```python
from build123d import *

# Parameters (mm, degrees)
SKETCH_1_R          = 2.1
SKETCH_1_R_2        = 4
SKETCH_1_R_3        = 11
EXTRUDE_1_DEPTH     = 3
SKETCH_3_R          = 2.1
CUT_EXTRUDE_1_DEPTH = 99.947101842
CHAMFER_2_SIZE      = 4
CHAMFER_3_SIZE      = 10
CHAMFER_3_SIZE2     = 7.354021529
SKETCH_4_W          = 7.6
SKETCH_4_H          = 9.2
CUT_EXTRUDE_2_DEPTH = 97.00692173
FILLET_1_R          = 2
SKETCH_5_R          = 2.1
CUT_EXTRUDE_3_DEPTH = 97.00692173
CHAMFER_1_SIZE      = 2
SKETCH_6_R          = 35
CUT_EXTRUDE_4_DEPTH = 97.00692173
FILLET_START        = -3
FILLET_2_DEPTH      = 6
CHAMFER_4_SIZE      = 4


with BuildPart() as part:
    # 草图1 → 凸台-拉伸1 (new, symmetric)
    with BuildSketch(Plane.XY):
        with BuildLine():
            Line((-55, 82.03370626), (-55, -2.96629374))
            Line((-55, -2.96629374), (-34.874074919, -2.96629374))
            ThreePointArc((-34.874074919, -2.96629374), (-7.334524273, -34.22286887), (30.595504664, -16.997502591))
            Line((30.595504664, -16.997502591), (52.449436567, 22.339574834))
            Line((52.449436567, 22.339574834), (-55, 82.03370626))
        make_face()
        with Locations((29, 0)):
            Circle(SKETCH_1_R, mode=Mode.SUBTRACT)
        with Locations((-14.5, -25.11473671)):
            Circle(SKETCH_1_R, mode=Mode.SUBTRACT)
        with Locations((-14.5, 25.11473671)):
            Circle(SKETCH_1_R, mode=Mode.SUBTRACT)
        with Locations((-9.625, 16.670989023)):
            Circle(SKETCH_1_R_2, mode=Mode.SUBTRACT)
        Circle(SKETCH_1_R_3, mode=Mode.SUBTRACT)
    extrude(amount=EXTRUDE_1_DEPTH, both=True)

    # 草图3 → 切除-拉伸1 (cut, through all)
    with BuildSketch(Plane.XY.offset(3)):
        with Locations((-45, 7.03370626)):
            Circle(SKETCH_3_R)
        with Locations((-45, 57.03370626)):
            Circle(SKETCH_3_R)
    extrude(amount=-CUT_EXTRUDE_1_DEPTH, mode=Mode.SUBTRACT)

    # 倒角2
    chamfer_2_edges = [part.edges().sort_by_distance(p)[0] for p in [
        (52.449436567, 22.339574834, 0),
        (-55, -2.96629374, 0),
    ]]
    chamfer(chamfer_2_edges, length=CHAMFER_2_SIZE)

    # 倒角3
    chamfer_3_edges = [part.edges().sort_by_distance(p)[0] for p in [
        (-55, 82.03370626, 0),
    ]]
    chamfer_3_side = [part.faces().sort_by_distance(p)[0] for p in [
        (-55, 41.53370626, 0),
    ]]
    chamfer(chamfer_3_edges, length=CHAMFER_3_SIZE, length2=CHAMFER_3_SIZE2, reference=chamfer_3_side[0])

    # 草图4 → 切除-拉伸2 (cut, through all)
    with BuildSketch(Plane.XY.offset(3)):
        with Locations((-18.5, 0)):
            Rectangle(SKETCH_4_W, SKETCH_4_H)
    extrude(amount=-CUT_EXTRUDE_2_DEPTH, mode=Mode.SUBTRACT)

    # 圆角1
    fillet_1_edges = [part.edges().sort_by_distance(p)[0] for p in [
        (-14.7, 4.6, 0),
        (-14.7, -4.6, 0),
        (-22.3, -4.6, 0),
        (-22.3, 4.6, 0),
    ]]
    fillet(fillet_1_edges, radius=FILLET_1_R)

    # 草图5 → 切除-拉伸3 (cut, through all)
    with BuildSketch(Plane.XY.offset(3)):
        with Locations((-4.856429312, 42.736577944)):
            Circle(SKETCH_5_R)
        with Locations((38.851434494, 18.454431385)):
            Circle(SKETCH_5_R)
    extrude(amount=-CUT_EXTRUDE_3_DEPTH, mode=Mode.SUBTRACT)

    # 倒角1
    chamfer_1_edges = [part.edges().sort_by_distance(p)[0] for p in [
        (-6.956429312, 42.736577944, 3),
        (36.751434494, 18.454431385, 3),
        (26.9, 0, 3),
        (-47.1, 7.03370626, 3),
        (-47.1, 57.03370626, 3),
    ]]
    chamfer(chamfer_1_edges, length=CHAMFER_1_SIZE)

    # 草图6 → 切除-拉伸4 (cut, through all)
    with BuildSketch(Plane.XY.offset(3)):
        Circle(SKETCH_6_R)
    extrude(amount=-CUT_EXTRUDE_4_DEPTH, mode=Mode.SUBTRACT)

    # 圆角2: read off the stored shape, not the designer's step
    # 圆角2 outline → 圆角2 (cut)
    with BuildSketch(Plane.XY.offset(FILLET_START)):
        with BuildLine():
            ThreePointArc((43.444408883, 6.130525003), (38.347542021, 3.611739847), (34.18941969, 7.488897201))
            ThreePointArc((34.18941969, 7.488897201), (34.62899868, -5.082563371), (30.595504664, -16.997502591))
            Line((30.595504664, -16.997502591), (43.444408883, 6.130525003))
        make_face()
    extrude(amount=FILLET_2_DEPTH, mode=Mode.SUBTRACT)

    # 倒角4
    # the kernel refuses this chamfer: 4, 3.699752538 mm, written as the material it takes off along each edge
    with BuildSketch(Plane(origin=(-34.874074919, -2.96629374, 13.286731952), x_dir=(-0.029279801283292956, 0.9995712547071425, 0), z_dir=(0, 0, -1))) as chamfer_4_piece_1:
        with BuildLine():
            Line((3.887831943, 0), (CHAMFER_4_SIZE * 0.0292798012833, -CHAMFER_4_SIZE * 0.999571254707))
            Line((CHAMFER_4_SIZE * 0.0292798012833, -CHAMFER_4_SIZE * 0.999571254707), (0, 0))
            ThreePointArc((0, 0), (1.998980438, -0.05398137), (3.887831943, 0))
        make_face()
    extrude(amount=26.573463904, mode=Mode.SUBTRACT)


solid = part.part
```
CAD build for the part. Positions are in the model's coordinates, mm. Round coordinates to 2 decimals unless told otherwise and drop trailing zeros. Write each loop counter-clockwise with the first axis right and the second up, starting at its lowest first coordinate (ties: lowest second). Pieces come first, ordered by that corner, then holes.
Item 1: Drill centre lines: L1, parallel to X at y = 20, z = 1.5; L2, parallel to X at y = 7, z = 2; L3, parallel to X at y = 22, z = -0.75. Where is each one in solid material? Low to high.
Filled in:
L1: x = -55 to -28.72, 28.72 to 36.76, 40.94 to 50.18
L2: x = -55 to -48.1, -41.9 to -34.29, 34.32 to 43.93
L3: x = -55 to -27.22, 27.22 to 49.6
Item 2: Band-saw the part on D-D on x = 31. Write the cut outline in (y, z).
Filled in:
outline: (16.25, -3) - (34.26, -3) - (34.26, 3) - (16.25, 3) - close
Item 3: Band-saw the part on B-B on z = -2. Write the cut outline in (x, y), then the cut area to 3 significant figures.
Filled in:
outline: (-55, 1.03) - (-51, -2.97) - (-38.87, -2.97) - (-34.99, 0.92) arc R35 cw to (34.19, 7.49) arc R5 ccw to (43.44, 6.13) - (50.51, 18.84) - (48.95, 24.28) - (-48.57, 78.46) - (-55, 72.03) - close; hole circle Ø4.2 at (-45, 7.03); hole circle Ø4.2 at (-45, 57.03); hole circle Ø4.2 at (-4.86, 42.74); hole circle Ø4.2 at (38.85, 18.45)
area: 3,470 mm2
Item 4: Band-saw the part on C-C on x = -30. Write the cut outline in (y, z).
Filled in:
outline: (18.03, -3) - (68.14, -3) - (68.14, 3) - (18.03, 3) - close
Item 5: Band-saw the part on A-A on x = -45. Write the cut outline in (y, z), then the cut area to 3 significant figures.
Filled in:
outline: (-2.97, -3) - (4.93, -3) - (4.93, 1) - (2.93, 3) - (-2.97, 3) - close; (9.13, -3) - (54.93, -3) - (54.93, 1) - (52.93, 3) - (11.13, 3) - (9.13, 1) - close; (59.13, -3) - (76.48, -3) - (76.48, 3) - (61.13, 3) - (59.13, 1) - close
area: 418 mm2
Item 6: Drop flat-ended pins along their axis: pin 1 Ø6.5 at (x, y) = (38.85, 18.45) entering from +Z; pin 2 Ø2 at (y, z) = (61.5, 1.5) entering from +X; pin 3 Ø1 at (x, z) = (-37.5, 0.5) entering from +Y; pin 4 Ø3.5 at (x, y) = (-45, 57.03) entering from -Z. Give the stop position or say it passes through.
Filled in:
pin 1: stops at z = 2.15
pin 2: stops at x = -16.24
pin 3: stops at y = 72.59
pin 4: passes through
Item 7: Mould opens along Y. For faces 1 (the flat face through (-51.741, 75.293, 0.042)), 2 (the cylindrical face through (38.43, 3.6, -0.04)), 3 (the conical face through (-42.94, 56.18, 1.13)), 4 (the conical face through (-5.34, 40.56, 1.13)) say: released by +Y, released by -Y, zero draft, split by the parting line, or undercut.
Filled in:
face 1: released by +Y
face 2: released by -Y
face 3: undercut
face 4: undercut
